For this review, take the finished solid that the model builds, in its own axes (mm). A direction names the side the tool comes from. Round coordinates to 2 decimals unless told otherwise and drop trailing zeros. Loops run counter-clockwise (first coordinate to the right, second up) from the corner with the lowest first, then second, coordinate; pieces in that order, holes last.
1) Mouldability with a two-part tool opening along Y and no side actions: class faces 3 (the flat face through (95.552, -6, -6)), 4 (the cylindrical face through (102.68, 6.79, 2.14)), 5 (the conical face through (16.075, -19.185, -14.71)) as pulls with the +Y half, pulls with the -Y half, needs draft (parallel to the pull), parting line crosses it, or undercut.
2) Tool access review of faces 1 (the conical face through (93.456, -27.202, 1.197)), 2 (the cylindrical face through (7.12, 6.79, 2.14)): name each direction out of +Z, -Z, +X, -X, +Y, -Y from which nothing blocks a thin tool from reaching the whole face with its end or side.
3) Insertion check: pin 1 (8 mm diameter, centred on y = 100.5, z = 112, fed in from -X); pin 2 (8 mm diameter, centred on x = 39.5, y = -153.5, fed in from +Z); pin 3 (1 mm diameter, centred on y = 160, z = -27.5, fed in from +X). Each pin has a flat end and moves straight along its axis. Give the tip position at first contact, or say it passes through.
4) Wall thickness on L1, parallel to X at y = -46, z = 193; L2, parallel to X at y = -60, z = 163.5; L3, parallel to Y at x = 9, z = 1.5: over which ranges is each line inside the solid? List them lowest first.
5) Take a section at A-A (y = 0). State the section outline as (x, z) points, then the cut area to 3 significant figures.
6) Take a section at C-C (x = 86). State the section outline as (y, z) points.
```python
from build123d import *

# Parameters (mm, degrees)
F0_W   = 14.447578
F0_H   = 7.120048
F0_W_2 = 40.552422
F0_H_2 = 6.468568


with BuildPart() as f1:
    # F0 (on Top) → F1 (revolve)
    with BuildSketch(Plane.XY):
        with Locations((7.223789, 3.560024)):
            Rectangle(F0_W, F0_H)
        with Locations((34.723789, 3.560024)):
            Rectangle(F0_W_2, F0_H)
        with Locations((75.276211, 3.560024)):
            Rectangle(F0_W_2, F0_H)
        with Locations((34.723789, 10.354332)):
            Rectangle(F0_W_2, F0_H_2)
        with Locations((102.776211, 3.560024)):
            Rectangle(F0_W, F0_H)
        with Locations((75.276211, 10.354332)):
            Rectangle(F0_W_2, F0_H_2)
        with BuildLine():
            Line((47.968432, 231.627907), (14.447578, 13.588616))
            Line((14.447578, 13.588616), (55, 13.588616))
            Line((55, 13.588616), (55, 230))
            ThreePointArc((55, 230), (51.391225, 230.412289), (47.968432, 231.627907))
        make_face()
        with BuildLine():
            Line((55, 230), (55, 13.588616))
            Line((55, 13.588616), (95.552422, 13.588616))
            Line((95.552422, 13.588616), (62.031568, 231.627907))
            ThreePointArc((62.031568, 231.627907), (58.608775, 230.412289), (55, 230))
        make_face()
        with BuildLine():
            ThreePointArc((55, 262), (39.412289, 249.608775), (47.968432, 231.627907))
            ThreePointArc((47.968432, 231.627907), (51.391225, 230.412289), (55, 230))
            Line((55, 230), (55, 262))
        make_face()
        with BuildLine():
            Line((55, 262), (55, 230))
            ThreePointArc((55, 230), (58.608775, 230.412289), (62.031568, 231.627907))
            ThreePointArc((62.031568, 231.627907), (68.573966, 237.529613), (71, 246))
            ThreePointArc((71, 246), (66.313708, 257.313708), (55, 262))
        make_face()
    revolve(axis=Axis((55, 0, 0), (1, 0, 0)))


solid = f1.part
```
Response:
1. face 3: needs draft
1. face 4: parting line crosses it
1. face 5: undercut
2. face 1: +X
2. face 2: -X
3. pin 1: stops at x = 34.88
3. pin 2: stops at z = 207.04
3. pin 3: stops at x = 72.76
4. L1: x = 42.86 to 67.14
4. L2: x = 39.13 to 70.87
4. L3: y = -6.96 to 6.96
5. outline: (0, -7.12) - (14.45, -7.12) - (14.45, -13.59) - (47.97, -231.63) arc R16 ccw to (55, -262) arc R16 ccw to (71, -246) arc R16 ccw to (62.03, -231.63) - (95.55, -13.59) - (95.55, -7.12) - (110, -7.12) - (110, 7.12) - (95.55, 7.12) - (95.55, 13.59) - (62.03, 231.63) arc R16 ccw to (71, 246) arc R16 ccw to (55, 262) arc R16 ccw to (47.97, 231.63) - (14.45, 13.59) - (14.45, 7.12) - (0, 7.12) - close
5. area: 24,900 mm2
6. outline: circle Ø151.45 at (0, 0)
